Geometry: final body of the model. Coordinates: model frame, mm. Face numbers are marked on the shaded views. A direction names the side the tool comes from. Round coordinates to 2 decimals unless told otherwise and drop trailing zeros. Write each loop counter-clockwise with the first axis right and the second up, starting at its lowest first coordinate (ties: lowest second). Pieces come first, ordered by that corner, then holes. Notation, with made-up numbers: M 57,64.5 L 84,64.5 A16 ccw 84,86.5 Z; hole C 85.25,16 d2. An arc over 180 degrees is marked long. Put each result on its own line as item: value. Start each with the question number.
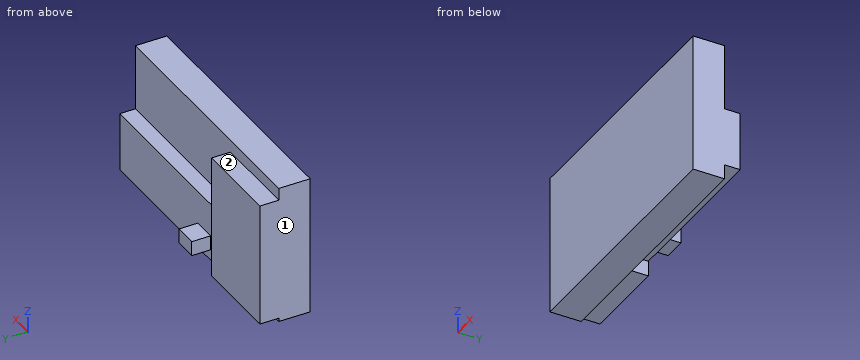
```python
from build123d import *

# Parameters (mm, degrees)
SKETCH1_W           = 82
SKETCH1_H           = 44.5
BOSS_EXTRUDE1_DEPTH = 10
SKETCH2_W           = 52.638055151
SKETCH2_H           = 18.722088721
BOSS_EXTRUDE2_DEPTH = 5
SKETCH3_W           = 27.641719578
SKETCH3_H           = 39.450206574
BOSS_EXTRUDE3_DEPTH = 6
SKETCH4_W           = 7.307754503
SKETCH4_H           = 4.667726012
BOSS_EXTRUDE4_DEPTH = 6


with BuildPart() as part:
    # Sketch1 → Boss-Extrude1 (new body)
    with BuildSketch(Plane(origin=(0, 0, 0), x_dir=(1, 0, 0), z_dir=(0, 1, 0))):
        with Locations((1.955938697, 0.340996169)):
            Rectangle(SKETCH1_W, SKETCH1_H)
    extrude(amount=BOSS_EXTRUDE1_DEPTH)

    # Sketch2 → Boss-Extrude2 (add)
    with BuildSketch(Plane(origin=(0, 10, 0), x_dir=(1, 0, 0), z_dir=(0, 1, 0))):
        with Locations((16.636911121, 8.563535134)):
            Rectangle(SKETCH2_W, SKETCH2_H)
    extrude(amount=BOSS_EXTRUDE2_DEPTH)

    # Sketch3 → Boss-Extrude3 (add)
    with BuildSketch(Plane(origin=(0, 10, 0), x_dir=(1, 0, 0), z_dir=(0, 1, 0))):
        with Locations((-25.223201514, 1.759430562)):
            Rectangle(SKETCH3_W, SKETCH3_H)
    extrude(amount=BOSS_EXTRUDE3_DEPTH)

    # Sketch4 → Boss-Extrude4 (add)
    with BuildSketch(Plane(origin=(0, 15, 0), x_dir=(1, 0, 0), z_dir=(0, 1, 0))):
        with Locations((-5.326444236, 12.169741761)):
            Rectangle(SKETCH4_W, SKETCH4_H)
    extrude(amount=BOSS_EXTRUDE4_DEPTH)


solid = part.part
```
1) Section A-A, the plane y = 13.25. Output: boundary loops of the cut face in (x, z), and give its area (3 significant figures).
2) Section D-D, the plane z = 11. Output: boundary loops of the cut face in (x, y).
3) Section B-B, the plane z = -2. Output: boundary loops of the cut face in (x, y), and give its area (3 significant figures).
4) Ray query, probe 1 along X at (y, z) = (13.75, -6); probe 2 along Z at (x, y) = (11.5, 13); probe 3 along X at (y, z) = (15.25, 11.5). Return the intervals inside material, ascending.
5) Section C-C, the plane x = 0. Output: boundary loops of the cut face in (y, z), and give its area (3 significant figures).
6) Access query for the marked faces 1 and 2. Directions: +Z, -Z, +X, -X, +Y, -Y. A direction counts if a zero-diameter tool reaches every point of the face in a straight line with its end or side. Return the directions, or none.
7) First-contact query: pin 1 (5.5 mm diameter, centred on x = 14, y = 12, fed in from +Z); pin 2 (2.5 mm diameter, centred on x = 20.5, y = 11.5, fed in from -Z); pin 3 (2 mm diameter, centred on x = 4, y = 17.5, fed in from +Z); pin 4 (15 mm diameter, centred on x = 21, z = -6, fed in from +Y). Flat tips, straight axial feed; report the tip coordinate or a pass-through.
Solved:
1. outline: M -39.04,-21.48 L -11.4,-21.48 L -11.4,17.97 L -39.04,17.97 Z; M -9.68,-17.92 L 42.96,-17.92 L 42.96,0.8 L -9.68,0.8 Z
1. area: 2,080 mm2
2. outline: M -39.04,0 L 42.96,0 L 42.96,10 L -11.4,10 L -11.4,16 L -39.04,16 Z
3. outline: M -39.04,0 L 42.96,0 L 42.96,15 L -9.68,15 L -9.68,10 L -11.4,10 L -11.4,16 L -39.04,16 Z
3. area: 1,250 mm2
4. probe 1: x = -39.04 to -11.4, -9.68 to 42.96
4. probe 2: z = -17.92 to 0.8
4. probe 3: x = -39.04 to -11.4
5. outline: M 0,-22.59 L 10,-22.59 L 10,-17.92 L 15,-17.92 L 15,0.8 L 10,0.8 L 10,21.91 L 0,21.91 Z
5. area: 539 mm2
6. face 1: +Z, -Z, -X, +Y, -Y
6. face 2: +Z, +X, -X, +Y
7. pin 1: stops at z = 21.91
7. pin 2: stops at z = -17.92
7. pin 3: passes through
7. pin 4: stops at y = 15
